```python
from build123d import *

# Parameters (mm, degrees)
BOSS_EXTRUDE1_DEPTH     = 10
SKETCH2_R               = 4
SKETCH2_R_2             = 4.5
SKETCH2_R_3             = 1.9
CUT_EXTRUDE1_DEPTH      = 11
CUT_EXTRUDE2_DEPTH      = 1
CUT_EXTRUDE2_DEPTH_BACK = 70
SKETCH5_W               = 1.016
SKETCH5_H               = 9.2075
CUT_EXTRUDE4_DEPTH      = 5
SKETCH6_W               = 12.35
SKETCH6_H               = 2.159
CUT_EXTRUDE5_DEPTH      = 9.954
SKETCH7_W               = 12.35
SKETCH7_H               = 2.159
CUT_EXTRUDE6_DEPTH      = 9.954


with BuildPart() as part:
    # Sketch1 → Boss-Extrude1 (new body)
    with BuildSketch(Plane.XY):
        Polygon((-34.5, 40.07390675), (34.5, 40.07390675), (34.5, -21.92609325), (13.861088822, -21.92609325), (13.861088822, -40.07390675), (-13.861088822, -40.07390675), (-13.861088822, -21.92609325), (-34.5, -21.92609325), align=None)
    extrude(amount=BOSS_EXTRUDE1_DEPTH)

    # Sketch2 → Cut-Extrude1 (cut, through all)
    with BuildSketch(Plane.XY.offset(10)):
        with Locations((0, -31)):
            Circle(SKETCH2_R)
        with Locations((0, -9)):
            Circle(SKETCH2_R_2)
        with Locations((0, -1)):
            Circle(SKETCH2_R_3)
        with Locations((8, -9)):
            Circle(SKETCH2_R_3)
        with Locations((0, -17)):
            Circle(SKETCH2_R_3)
        with Locations((-8, -9)):
            Circle(SKETCH2_R_3)
    extrude(amount=-CUT_EXTRUDE1_DEPTH, mode=Mode.SUBTRACT)

    # Sketch4 → Cut-Extrude2 (cut, two sides)
    with BuildSketch(Plane.ZY.offset(34.5)) as cut_extrude2_sk:
        Polygon((5, 210.681154515), (5, 40.07390675), (5, 20.97390675), (10, 20.97390675), (180.607247765, 20.97390675), (431.008352756, 252.763937984), (255.401104991, 442.471185749), align=None)
    extrude(amount=CUT_EXTRUDE2_DEPTH, mode=Mode.SUBTRACT)
    extrude(cut_extrude2_sk.sketch, amount=-CUT_EXTRUDE2_DEPTH_BACK, mode=Mode.SUBTRACT)

    # Sketch5 → Cut-Extrude4 (cut)
    with BuildSketch(Plane.XY.offset(10)):
        with Locations((0, 16.37015675)):
            Rectangle(SKETCH5_W, SKETCH5_H)
    extrude(amount=-CUT_EXTRUDE4_DEPTH, mode=Mode.SUBTRACT)

    # Sketch6 → Cut-Extrude5 (cut)
    with BuildSketch(Plane(origin=(0, 20.97390675, 0), x_dir=(1, 0, 0), z_dir=(0, 1, 0))):
        with Locations((-6.683, -6.0795)):
            Rectangle(SKETCH6_W, SKETCH6_H)
    extrude(amount=-CUT_EXTRUDE5_DEPTH, mode=Mode.SUBTRACT)

    # Sketch7 → Cut-Extrude6 (cut)
    with BuildSketch(Plane(origin=(0, 20.97390675, 0), x_dir=(1, 0, 0), z_dir=(0, 1, 0))):
        with Locations((6.683, -6.0795)):
            Rectangle(SKETCH7_W, SKETCH7_H)
    extrude(amount=-CUT_EXTRUDE6_DEPTH, mode=Mode.SUBTRACT)


solid = part.part
```
CAD build for the part. Positions are in the model's coordinates, mm. A direction names the side the tool comes from. Round coordinates to 2 decimals unless told otherwise and drop trailing zeros. Write each loop counter-clockwise with the first axis right and the second up, starting at its lowest first coordinate (ties: lowest second). Pieces come first, ordered by that corner, then holes. Notation, with made-up numbers: (-37.5, 48) - (-21.5, 48) arc R27 ccw to (-21.5, 87) - close; hole circle Ø11 at (-22, -15.75). An arc over 180 degrees is marked (long way). Return JSON: item names as keys, results as strings. Group by question number.
Item 1: Probe probe 1 along Y at (x, z) = (0, 2); probe 2 along Y at (x, z) = (0, 5.5); probe 3 along Z at (x, y) = (7, 15). List the from-to ranges inside material, lowest first.
Item 2: Mould opens along Y. For faces 1 (the face through (-7, 16, 7.159)), 2 (the face through (-9.508, -10.156, 5.07)), 3 (the face through (-0.247, -15.116, 5.07)), 4 (the face through (-7, 11.02, 6)) say: +Y half, -Y half, draft (parallel to the pull), parting line (faces both ways), or undercut.
Item 3: 3-axis set-ups, long thin cutter, end or side, ignore diameter. For faces 5 (the face through (21, 20.974, 7)), 6 (the face through (-0.508, 16, 9)), 7 (the face through (-0.521, -27.034, 5.07)), 8 (the face through (7, 16, 7.159)), 9 (the face through (-24, -21.926, 5)): which of +Z, -Z, +X, -X, +Y, -Y reach the whole face in a straight line?
Item 4: Band-saw the part on D-D on x = 26. List the corners of the cut face in (y, z), plus the area to 4 significant figures.
Item 5: Band-saw the part on C-C on z = 1.25. List the corners of the cut face in (x, y).
Item 6: Band-saw the part on B-B on x = -8. List the corners of the cut face in (y, z), plus the area to 3 significant figures.
Item 7: Band-saw the part on A-A on y = -17. List the corners of the cut face in (x, z), plus the area to 3 significant figures.
Item 8: Flat gauge pins, fed straight in: pin 1 Ø0.8 at (x, z) = (0, 8) entering from +Y; pin 2 Ø5 at (x, z) = (-19.5, 3.5) entering from -Y; pin 3 Ø8 at (x, y) = (0, -9) entering from +Z; pin 4 Ø5 at (y, z) = (-29.5, 6) entering from +X. Where does each tip first touch, or does it go through?
Resolved:
{
 "1": {"probe 1": "y = -40.07 to -35, -27 to -18.9, -15.1 to -13.5, -4.5 to -2.9, 0.9 to 40.07", "probe 2": "y = -40.07 to -35, -27 to -18.9, -15.1 to -13.5, -4.5 to -2.9, 0.9 to 11.77", "probe 3": "z = 0 to 5, 7.16 to 10"},
 "2": {"face 1": "draft", "face 2": "undercut", "face 3": "undercut", "face 4": "+Y half"},
 "3": {"face 5": "+Z, +X, -X, +Y", "face 6": "+Z, +Y", "face 7": "+Z, -Z", "face 8": "+Y", "face 9": "+Z, -Z, -X, -Y"},
 "4": {"outline": "(-21.93, 0) - (40.07, 0) - (40.07, 5) - (20.97, 5) - (20.97, 10) - (-21.93, 10) - close", "area": "524.5 mm²"},
 "5": {"outline": "(-34.5, -21.93) - (-13.86, -21.93) - (-13.86, -40.07) - (13.86, -40.07) - (13.86, -21.93) - (34.5, -21.93) - (34.5, 40.07) - (-34.5, 40.07) - close; hole circle Ø3.8 at (-8, -9); hole circle Ø9 at (0, -9); hole circle Ø8 at (0, -31); hole circle Ø3.8 at (0, -17); hole circle Ø3.8 at (0, -1); hole circle Ø3.8 at (8, -9)"},
 "6": {"outline": "(-40.07, 0) - (-10.9, 0) - (-10.9, 10) - (-40.07, 10) - close; (-7.1, 0) - (40.07, 0) - (40.07, 5) - (11.02, 5) - (11.02, 7.16) - (20.97, 7.16) - (20.97, 10) - (-7.1, 10) - close", "area": "646 mm²"},
 "7": {"outline": "(-34.5, 0) - (-1.9, 0) - (-1.9, 10) - (-34.5, 10) - close; (1.9, 0) - (34.5, 0) - (34.5, 10) - (1.9, 10) - close", "area": "652 mm²"},
 "8": {"pin 1": "stops at y = 11.77", "pin 2": "stops at y = -21.93", "pin 3": "passes through", "pin 4": "stops at x = 13.86"}
}
